Input: part model. Units: mm. Frame: model coordinates. Face numbers are marked on the shaded views. A direction names the side the tool comes from. Give positions to 0.01 mm unless a question says otherwise; leave off trailing zeros. Loops run counter-clockwise (first coordinate to the right, second up) from the corner with the lowest first, then second, coordinate; pieces in that order, holes last. Notation, with made-up numbers: M 39.5,31.5 L 55.5,31.5 A38 cw 55.5,70.5 Z; hole C 74,41 d2. An arc over 180 degrees is marked long. Answer as a JSON object with one key per item and string values. Group by question number.
1) Access query for the marked faces 1 and 2. Directions: +Z, -Z, +X, -X, +Y, -Y. A direction counts if a zero-diameter tool reaches every point of the face in a straight line with its end or side. Return the directions, or none.
2) First-contact query: P1, Ø3.5, axis at x = 5.5, y = 5, coming from the +Z side; P2, Ø0.6, axis at x = -6.5, z = 9, coming from the -Y side. Flat tips, straight axial feed; report the tip coordinate or a pass-through.
3) Section query C-C on z = 9.5. Return loops of the section in (x, y).
4) Section query A-A on x = -5. Return loops of the section in (y, z).
5) Section query B-B on y = 7. Return loops of the section in (x, z).
6) Ray query, L1, parallel to Z at x = -8, y = 11.5; L2, parallel to Z at x = 8.5, y = 26. Return the intervals inside material, ascending.
from build123d import *

# Parameters (mm, degrees)
SALIENTE_EXTRUIR1_DEPTH      = 16
SALIENTE_EXTRUIR1_DEPTH_BACK = 16


with BuildPart() as part:
    # Croquis1 → Saliente-Extruir1 (new, two sides: drawn at the far end of the back side and taken through both)
    with BuildSketch(Plane(origin=(0, 0, 0), x_dir=(0, 0, -1), z_dir=(1, 0, 0)).offset(-SALIENTE_EXTRUIR1_DEPTH_BACK)):
        Polygon((0, 0), (0, 32), (-7.320508076, 32), (-10, 22), (-10, 12), (-8, 12), (-8, 0), align=None)
    extrude(amount=SALIENTE_EXTRUIR1_DEPTH + SALIENTE_EXTRUIR1_DEPTH_BACK)


solid = part.part
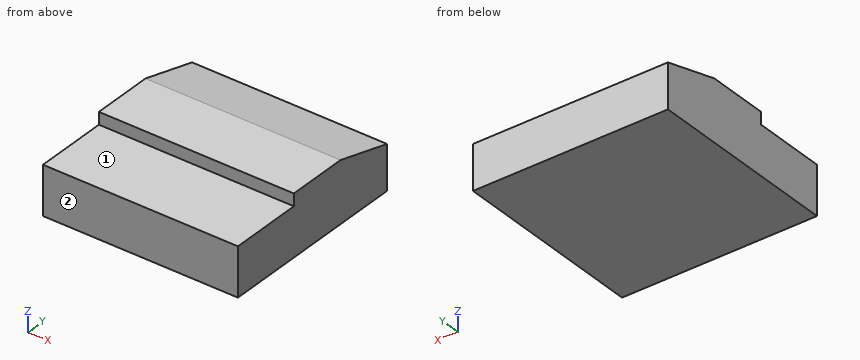
Output:
{
 "1": {"face 1": "+Z, +X, -X, -Y", "face 2": "+Z, -Z, +X, -X, -Y"},
 "2": {"P1": "stops at z = 8", "P2": "stops at y = 12"},
 "3": {"outline": "M -16,12 L 16,12 L 16,23.87 L -16,23.87 Z"},
 "4": {"outline": "M 0,0 L 32,0 L 32,7.32 L 22,10 L 12,10 L 12,8 L 0,8 Z"},
 "5": {"outline": "M -16,0 L 16,0 L 16,8 L -16,8 Z"},
 "6": {"L1": "z = 0 to 8", "L2": "z = 0 to 8.93"}
}
